Here's how the part is built. I have some questions about the finished solid (model axes, mm). Face numbers are marked on the shaded views. A direction names the side the tool comes from. Give positions to 0.01 mm unless a question says otherwise; leave off trailing zeros. Write each loop counter-clockwise with the first axis right and the second up, starting at its lowest first coordinate (ties: lowest second). Pieces come first, ordered by that corner, then holes. Notation, with made-up numbers: (66.5, -23) - (123.5, -23) arc R22 ccw to (123.5, 0) - close; hole circle Ø3 at (3.5, 69.25). An arc over 180 degrees is marked (long way). Write each question's results on one line, items separated by ' | '. Start each with the question number.
Item 1: Will these pins go through, and if not, where does the flat tip stop? P1, Ø2.5, axis at x = 12.5, z = -17.5, coming from the +Y side (3 decimals); P2, Ø8.5, axis at x = 12.7, z = -17.78, coming from the -Y side (3 decimals); P3, Ø1, axis at y = -66.5, z = -19, coming from the +X side (3 decimals).
Item 2: We'd pull the mould along Y, two halves only. Please class the marked faces 1, 2 and 3: +Y half, -Y half, draft (parallel to the pull), parting line (faces both ways), or undercut.
Item 3: Suppose I cut it at C-C on x = -24. List the corners of the cut face in (y, z) for me (3 decimals).
Item 4: Which directions (+Z, -Z, +X, -X, +Y, -Y) give clear straight access to the entire face, cutting with the end or side of a thin tool? Please do the marked faces 4 and 5.
Item 5: Please list where these lines run through material, in increasing order: line 1 along Y through (x, z) = (13, -25.75) (3 decimals); line 2 along X through (y, z) = (122.4, -17.78); line 3 along X through (y, z) = (16, -26.75) (3 decimals).
Item 6: Suppose I cut it at A-A on y = -60. List the corners of the cut face in (x, z) for me (3 decimals), then the cut area to 3 significant figures.
Item 7: Suppose I cut it at B-B on z = -25.4. List the corners of the cut face in (x, y) for me (3 decimals).
```python
from build123d import *

# Parameters (mm, degrees)
BOSS_EXTRUDE1_DEPTH   = 123.825
SKETCH2_W             = 22.86
SKETCH2_H             = 3.683
BOSS_EXTRUDE2_DEPTH   = 24.13
SKETCH8_R             = 2.667
CUT_EXTRUDE3_DEPTH    = 5.08
SKETCH3_R             = 3.048
CUT_EXTRUDE1_DEPTH    = 2.54
F_3_0MM_DOWEL_HOLE1_D = 3
SKETCH6_W             = 60.494674014
SKETCH6_H             = 234.95
CUT_EXTRUDE2_DEPTH    = 19.05
SKETCH7_W             = 6.35
SKETCH7_H             = 18.890851128
BOSS_EXTRUDE3_DEPTH   = 234.95
FILLET1_R             = 2.54


with BuildPart() as part:
    # Sketch1 → Boss-Extrude1 (new, symmetric)
    with BuildSketch(Plane(origin=(0, 0, 0), x_dir=(1, 0, 0), z_dir=(0, 1, 0))):
        with BuildLine():
            ThreePointArc((30.247337007, 9.652), (0, 31.75), (-30.247337007, 9.652))
            Line((-30.247337007, 9.652), (30.247337007, 9.652))
        make_face()
    extrude(amount=BOSS_EXTRUDE1_DEPTH, both=True)

    # Sketch2 → Boss-Extrude2 (add)
    with BuildSketch(Plane.XZ.offset(123.825)):
        with Locations((0, -11.4935)):
            Rectangle(SKETCH2_W, SKETCH2_H)
    extrude(amount=BOSS_EXTRUDE2_DEPTH)

    # Sketch8 → Cut-Extrude3 (cut)
    with BuildSketch(Plane(origin=(0, 123.825, 0), x_dir=(1, 0, 0), z_dir=(0, 1, 0))):
        with Locations(Location((0, 25.4, 0), (0, 0, 270))):
            Circle(SKETCH8_R)
        with Locations(Location((-12.7, 17.78, 0), (0, 0, 270))):
            Circle(SKETCH8_R)
        with Locations(Location((12.7, 17.78, 0), (0, 0, 270))):
            Circle(SKETCH8_R)
    extrude(amount=-CUT_EXTRUDE3_DEPTH, mode=Mode.SUBTRACT)

    # Sketch3 → Cut-Extrude1 (cut)
    with BuildSketch(Plane.XY.offset(-9.652)):
        with Locations((0, -130.316247378)):
            Circle(SKETCH3_R)
        with Locations((-7.62, -143.514474532)):
            Circle(SKETCH3_R)
        with Locations((7.62, -143.514474532)):
            Circle(SKETCH3_R)
    extrude(amount=-CUT_EXTRUDE1_DEPTH, mode=Mode.SUBTRACT)

    # Ø3.0mm Dowel Hole1 (through all)
    with Locations(Plane.XY.offset(-9.652)):
        with Locations((0, -130.316247378), (7.62, -143.514474532), (-7.62, -143.514474532)):
            Hole(F_3_0MM_DOWEL_HOLE1_D / 2)

    # Sketch6 → Cut-Extrude2 (cut)
    with BuildSketch(Plane(origin=(0, 0, -31.75), x_dir=(-1, 0, 0), z_dir=(0, 0, -1))):
        Rectangle(SKETCH6_W, SKETCH6_H)
    extrude(amount=-CUT_EXTRUDE2_DEPTH, mode=Mode.SUBTRACT)

    # Sketch7 → Boss-Extrude3 (add)
    with BuildSketch(Plane.XZ.offset(-117.475)):
        with BuildLine():
            ThreePointArc((-3.175, -31.590851128), (0, -31.75), (3.175, -31.590851128))
            Line((3.175, -31.590851128), (-3.175, -31.590851128))
        make_face()
        with Locations((0, -22.145425564)):
            Rectangle(SKETCH7_W, SKETCH7_H)
    extrude(amount=BOSS_EXTRUDE3_DEPTH)

    # Fillet1
    # the kernel refuses this fillet: 2.54 mm, written as the material it adds along each edge
    with BuildSketch(Plane(origin=(3.175, 117.475, -37.940851128), x_dir=(1, 0, 0), z_dir=(0, 0, 1))) as fillet1_piece_1_section:
        with BuildLine():
            CenterArc((FILLET1_R, -FILLET1_R), FILLET1_R, 90, 90)
            Line((0, -FILLET1_R), (0, 0))
            Line((0, 0), (FILLET1_R, 0))
        make_face()
    fillet1_piece_1 = extrude(amount=25.240851128, mode=Mode.PRIVATE)
    fillet1_piece_1 = fillet1_piece_1 & Plane(origin=(0, 116.898787332, 0), x_dir=(0.9526720317087093, 0, -0.3040000000000001), z_dir=(0, 1, 0)) * Cylinder(31.75, 61, mode=Mode.PRIVATE)
    add(fillet1_piece_1)
    with BuildSketch(Plane(origin=(3.175, -117.475, -37.940851128), x_dir=(1, 0, 0), z_dir=(0, 0, 1))) as fillet1_piece_2_section:
        with BuildLine():
            CenterArc((FILLET1_R, FILLET1_R), FILLET1_R, 180, 90)
            Line((0, FILLET1_R), (0, 0))
            Line((0, 0), (FILLET1_R, 0))
        make_face()
    fillet1_piece_2 = extrude(amount=25.240851128, mode=Mode.PRIVATE)
    fillet1_piece_2 = fillet1_piece_2 & Plane(origin=(0, -116.898787332, 0), x_dir=(0.9526720317087093, 0, -0.3040000000000001), z_dir=(0, 1, 0)) * Cylinder(31.75, 61, mode=Mode.PRIVATE)
    add(fillet1_piece_2)
    with BuildSketch(Plane(origin=(-3.175, 117.475, -12.7), x_dir=(-1, 0, 0), z_dir=(0, 0, -1))) as fillet1_piece_3_section:
        with BuildLine():
            CenterArc((FILLET1_R, -FILLET1_R), FILLET1_R, 90, 90)
            Line((0, -FILLET1_R), (0, 0))
            Line((0, 0), (FILLET1_R, 0))
        make_face()
    fillet1_piece_3 = extrude(amount=25.240851128, mode=Mode.PRIVATE)
    fillet1_piece_3 = fillet1_piece_3 & Plane(origin=(0, 116.898782869, 0), x_dir=(0.9526720317087093, 0, -0.3040000000000001), z_dir=(0, 1, 0)) * Cylinder(31.75, 61, mode=Mode.PRIVATE)
    add(fillet1_piece_3)
    with BuildSketch(Plane(origin=(-3.175, -117.475, -12.7), x_dir=(-1, 0, 0), z_dir=(0, 0, -1))) as fillet1_piece_4_section:
        with BuildLine():
            CenterArc((FILLET1_R, FILLET1_R), FILLET1_R, 180, 90)
            Line((0, FILLET1_R), (0, 0))
            Line((0, 0), (FILLET1_R, 0))
        make_face()
    fillet1_piece_4 = extrude(amount=25.240851128, mode=Mode.PRIVATE)
    fillet1_piece_4 = fillet1_piece_4 & Plane(origin=(0, -116.898782869, 0), x_dir=(0.9526720317087093, 0, -0.3040000000000001), z_dir=(0, 1, 0)) * Cylinder(31.75, 61, mode=Mode.PRIVATE)
    add(fillet1_piece_4)
    with BuildSketch(Plane(origin=(-3.175, 123.825, -12.7), x_dir=(-1, 0, 0), z_dir=(0, -1, 0))) as fillet1_piece_5:
        with BuildLine():
            CenterArc((FILLET1_R, FILLET1_R), FILLET1_R, 180, 90)
            Line((0, FILLET1_R), (0, 0))
            Line((0, 0), (FILLET1_R, 0))
        make_face()
    extrude(amount=247.65)
    with BuildSketch(Plane(origin=(3.175, 123.825, -12.7), x_dir=(1, 0, 0), z_dir=(0, -1, 0))) as fillet1_piece_6:
        with BuildLine():
            CenterArc((FILLET1_R, -FILLET1_R), FILLET1_R, 90, 90)
            Line((0, -FILLET1_R), (0, 0))
            Line((0, 0), (FILLET1_R, 0))
        make_face()
    extrude(amount=247.65)


solid = part.part
```
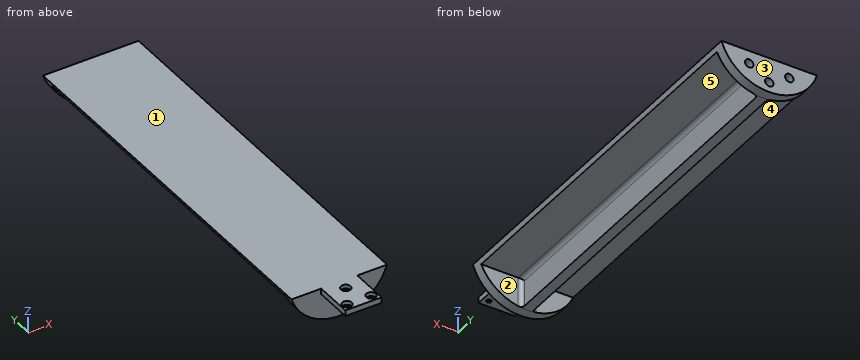
Checked values:
1) P1: stops at y = 118.745 | P2: stops at y = -123.825 | P3: stops at x = 3.175
2) face 1: draft | face 2: undercut | face 3: +Y half
3) outline: (-123.825, -20.786) - (-117.475, -20.786) - (-117.475, -12.7) - (117.475, -12.7) - (117.475, -20.786) - (123.825, -20.786) - (123.825, -9.652) - (-123.825, -9.652) - close
4) face 4: -Z, -X | face 5: -Z, +X
5) line 1: y = -123.825 to -117.475, 117.475 to 123.825 | line 2: x = -26.3 to -15.37, -10.03 to 10.03, 15.37 to 26.3 | line 3: x = -3.175 to 3.175
6) outline: (-30.247, -9.652) arc R31.75 ccw to (-29.099, -12.7) - (-5.715, -12.7) arc R2.54 cw to (-3.175, -15.24) - (-3.175, -31.591) arc R31.75 ccw to (3.175, -31.591) - (3.175, -15.24) arc R2.54 cw to (5.715, -12.7) - (29.099, -12.7) arc R31.75 ccw to (30.247, -9.652) - close | area: 304 mm^2
7) outline: (-19.05, -123.825) - (19.05, -123.825) - (19.05, -117.475) - (5.715, -117.475) arc R2.54 cw to (3.175, -114.935) - (3.175, 114.935) arc R2.54 cw to (5.715, 117.475) - (19.05, 117.475) - (19.05, 123.825) - (2.667, 123.825) - (2.667, 118.745) - (-2.667, 118.745) - (-2.667, 123.825) - (-19.05, 123.825) - (-19.05, 117.475) - (-5.715, 117.475) arc R2.54 cw to (-3.175, 114.935) - (-3.175, -114.935) arc R2.54 cw to (-5.715, -117.475) - (-19.05, -117.475) - close
